Model file for the job. Use its own axes, mm. A direction names the side the tool comes from. Round coordinates to 2 decimals unless told otherwise and drop trailing zeros. Order: outer loops, then holes, each group sorted by start corner. A loop starts at its lowest first (then second) coordinate and runs counter-clockwise, first axis right, second up. Notation, with made-up numbers: (-22, -38) - (20, -38) arc R35 ccw to (20, -2) - close; hole circle Ø7 at (-10, 73). An arc over 180 degrees is marked (long way). Put each result on its own line as item: value. Start each with the question number.
Item 1: Saw through at D-D on x = 108. List the corners of the cut face in (y, z).
Item 2: Saw through at B-B on y = 119.5. List the corners of the cut face in (x, z), plus the area to 3 significant figures.
Item 3: Saw through at A-A on x = 43. List the corners of the cut face in (y, z).
Item 4: Probe probe 1 along X at (y, z) = (160, 5.15); probe 2 along Y at (x, z) = (22.5, 5); probe 3 along X at (y, z) = (115.5, 4.75). List the from-to ranges inside material, lowest first.
Item 5: Which spindle directions (+Z, -Z, +X, -X, +Y, -Y) get a long thin tool onto all of the face, cutting with end or side? Do faces 1 (the face through (187.632, 219.024, -3.916)), 2 (the face through (44, 145.811, 3)), 3 (the face through (153, 240, 3)). Say none if no direction does.
Item 6: Saw through at C-C on z = -6.25. List the corners of the cut face in (x, y).
Item 7: Pin check, flat tips, straight feed: pin 1 Ø1.5 at (x, z) = (307.5, 2) entering from +Y; pin 2 Ø1.5 at (y, z) = (238, 2.5) entering from -X; pin 3 Ø4 at (x, z) = (2.5, 3.5) entering from -Y; pin 4 Ø4.5 at (x, y) = (100, 100) entering from +Z. Stop position of each tip, or through.
Item 8: Mould opens along X. For faces 4 (the face through (218.675, 181.627, -4.93)), 5 (the face through (153, 40, 3)), 6 (the face through (119.08, 100.56, 3.97)) say: pulls with the +X half, pulls with the -X half, needs draft (parallel to the pull), parting line crosses it, or undercut.
Autodesk Fusion 360 part; units mm, degrees
sketch "Skizze1" plane through (0, 0, 0) normal (0, 0, 1) x (1, 0, 0)
  line L0 (0, 0) -> (240, 0)
  line L1 (240, 0) -> (240, 240)
  line L2 (240, 240) -> (0, 240)
  line L3 (0, 240) -> (0, 0)
  dimension "d1" = 240
  dimension "d2" = 240
extrude "Extrusion1" add sketch "Skizze1" along normal blind 6
sketch "Skizze2" plane through (0, 0, 6) normal (0, 0, 1) x (-1, 0, 0)
  line L0 (0, -240) -> (0, 0)
  line L1 (0, 0) -> (-240, 0)
  line L2 (-240, 0) -> (-240, -240)
  line L3 (-240, -240) -> (0, -240)
  circle A0 centre (-150, -160) radius 70
  dimension "d6" = 140
extrude "Extrusion2" cut sketch "Skizze2" against normal blind 2 contours A0
sketch "Skizze3" plane through (0, 0, 4) normal (0, 0, 1) x (-1, 0, 0)
  circle A0 centre (-150, -160) radius 70
  circle A1 centre (-150, -160) radius 67
  dimension "d9" = 134
extrude "Extrusion3" cut sketch "Skizze3" against normal blind 35 contours A1
extrude "Extrusion4" add 1 faces at (208.7542, 124.1511, 4) along direction (0, 0, 1) blind 2
sketch "Skizze4" plane through (0, 0, 0) normal (0, 0, -1) x (1, 0, 0)
  circle A0 centre (150, -160) radius 67
  line L0 (0, 0) -> (0, -240)
  line L1 (0, -240) -> (240, -240)
  line L2 (240, -240) -> (240, 0)
  line L3 (240, 0) -> (0, 0)
  circle A1 centre (150, -160) radius 70
  dimension "d14" = 140
extrude "Extrusion5" cut sketch "Skizze4" against normal blind 2 contours A1
extrude "Extrusion6" cut 1 faces at (80, 0, 2) along direction (0, 1, 0) blind 40
sketch "Skizze5" plane through (0, 0, 0) normal (0, 0, -1) x (1, 0, 0)
  line L0 (240, -40) -> (0, -40)
  line L1 (0, -40) -> (0, -240)
  line L2 (0, -240) -> (240, -240)
  line L3 (240, -240) -> (240, -40)
  circle A0 centre (150, -160) radius 70
  circle A1 centre (150, -160) radius 70
  circle A2 centre (150, -160) radius 72
  dimension "d19" = 144
extrude "Extrusion7" add sketch "Skizze5" along normal blind 10 contours A2
extrude "Extrusion8" add 1 faces at (240, 106.6667, 4) along direction (1, 0, 0) blind 70
sketch "Skizze6" plane through (0, 0, 0) normal (0, 0, -1) x (1, 0, 0)
  circle A0 centre (150, -160) radius 72
  line L0 (310, -40) -> (0, -40)
  line L1 (0, -40) -> (0, -240)
  line L2 (0, -240) -> (310, -240)
  line L3 (310, -240) -> (310, -40)
  line L4 (0, -40) -> (5, -40)
  line L5 (5, -40) -> (5, -45)
  line L6 (5, -45) -> (0, -45)
  line L7 (0, -45) -> (0, -40)
  line L8 (0, -240) -> (5, -240)
  line L9 (5, -240) -> (5, -235)
  line L10 (5, -235) -> (0, -235)
  line L11 (0, -235) -> (0, -240)
  line L12 (310, -240) -> (305, -240)
  line L13 (305, -240) -> (305, -235)
  line L14 (305, -235) -> (310, -235)
  line L15 (310, -235) -> (310, -240)
  line L16 (310, -40) -> (305, -40)
  line L17 (305, -40) -> (305, -45)
  line L18 (305, -45) -> (310, -45)
  line L19 (310, -45) -> (310, -40)
  dimension "d24" = 5
  dimension "d25" = 5
extrude "Extrusion9" cut sketch "Skizze6" against normal blind 20 contours L0 L3 L16 L17 L18 L19 | L0 L1 L4 L5 L6 L7 | L2 L3 L12 L13 L14 L15 | L1 L2 L8 L9 L10 L11
sketch "Skizze7" plane through (0, 0, 0) normal (0, 0, -1) x (1, 0, 0)
  circle A0 centre (150, -160) radius 72
  line L0 (305, -240) -> (305, -235)
  line L1 (305, -235) -> (310, -235)
  line L2 (310, -235) -> (310, -45)
  line L3 (310, -45) -> (305, -45)
  line L4 (305, -45) -> (305, -40)
  line L5 (305, -40) -> (5, -40)
  line L6 (5, -40) -> (5, -45)
  line L7 (5, -45) -> (0, -45)
  line L8 (0, -45) -> (0, -235)
  line L9 (0, -235) -> (5, -235)
  line L10 (5, -235) -> (5, -240)
  line L11 (5, -240) -> (305, -240)
  line L12 (18.5416, -65.8113) -> (68.5416, -65.8113)
  line L13 (68.5416, -65.8113) -> (68.5416, -145.8113)
  line L14 (68.5416, -145.8113) -> (18.5416, -145.8113)
  line L15 (18.5416, -145.8113) -> (18.5416, -65.8113)
  circle A1 centre (64.5928, -155.8111) radius 2
  circle A2 centre (22.0928, -155.8111) radius 2
  circle A3 centre (64.5928, -55.1368) radius 2
  circle A4 centre (22.0928, -55.1368) radius 2
  dimension "d28" = 80
  dimension "d29" = 42.5
  dimension "d30" = 4
  dimension "d31" = 4
  dimension "d32" = 4
  dimension "d33" = 4
extrude "Extrusion10" cut sketch "Skizze7" against normal blind 90 contours L12 L13 L14 L15 | A1 | A2 | A3 | A4
sketch "Skizze8" plane through (0, 0, 6) normal (0, 0, 1) x (-1, 0, 0)
  line L0 (-68.5416, -145.8113) -> (-68.5416, -65.8113)
  line L1 (-68.5416, -65.8113) -> (-18.5416, -65.8113)
  line L2 (-18.5416, -65.8113) -> (-18.5416, -145.8113)
  line L3 (-18.5416, -145.8113) -> (-68.5416, -145.8113)
  circle A0 centre (-64.5928, -155.8111) radius 2
  circle A1 centre (-64.5928, -55.1368) radius 2
  circle A2 centre (-22.0928, -155.8111) radius 2
  circle A3 centre (-22.0928, -55.1368) radius 2
  circle A4 centre (-150, -160) radius 67
  line L4 (-310, -235) -> (-305, -235)
  line L5 (-305, -235) -> (-305, -240)
  line L6 (-305, -240) -> (-5, -240)
  line L7 (-5, -240) -> (-5, -235)
  line L8 (-5, -235) -> (0, -235)
  line L9 (0, -235) -> (0, -45)
  line L10 (0, -45) -> (-5, -45)
  line L11 (-5, -45) -> (-5, -40)
  line L12 (-5, -40) -> (-305, -40)
  line L13 (-305, -40) -> (-305, -45)
  line L14 (-305, -45) -> (-310, -45)
  line L15 (-310, -45) -> (-310, -235)
  circle A5 centre (-100, -225) radius 2
  circle A6 centre (-200, -225) radius 2
  circle A7 centre (-200, -100) radius 2
  circle A8 centre (-100, -100) radius 2
  dimension "d36" = 4
  dimension "d37" = 4
  dimension "d38" = 4
  dimension "d39" = 4
extrude "Extrusion11" cut sketch "Skizze8" against normal blind 3 contours A5 | A6 | A7 | A8
Results found:
1. outline: (40, 0) - (101.52, 0) - (101.52, -10) - (104, -10) - (104, 2) - (107.8, 2) - (107.8, 6) - (40, 6) - close; (212.2, 2) - (216, 2) - (216, -10) - (218.48, -10) - (218.48, 0) - (240, 0) - (240, 6) - (212.2, 6) - close
2. outline: (0, 0) - (18.54, 0) - (18.54, 6) - (0, 6) - close; (68.54, 0) - (90.47, 0) - (90.47, -10) - (92.91, -10) - (92.91, 2) - (96.63, 2) - (96.63, 6) - (68.54, 6) - close; (203.37, 2) - (207.09, 2) - (207.09, -10) - (209.53, -10) - (209.53, 0) - (310, 0) - (310, 6) - (203.37, 6) - close
2. area: 953 mm²
3. outline: (40, 0) - (65.81, 0) - (65.81, 6) - (40, 6) - close; (145.81, 0) - (240, 0) - (240, 6) - (145.81, 6) - close
4. probe 1: x = 0 to 83, 217 to 310
4. probe 2: y = 40 to 53.18, 57.09 to 65.81, 145.81 to 153.85, 157.77 to 240
4. probe 3: x = 0 to 18.54, 68.54 to 99.91, 200.09 to 310
5. face 1: -Z
5. face 2: +Z, -Z
5. face 3: +Z, -Z, +X, -X, +Y
6. outline: circle Ø144 at (150, 160); hole circle Ø140 at (150, 160)
7. pin 1: stops at y = 235
7. pin 2: stops at x = 5
7. pin 3: stops at y = 45
7. pin 4: stops at z = 6
8. face 4: parting line crosses it
8. face 5: needs draft
8. face 6: undercut
